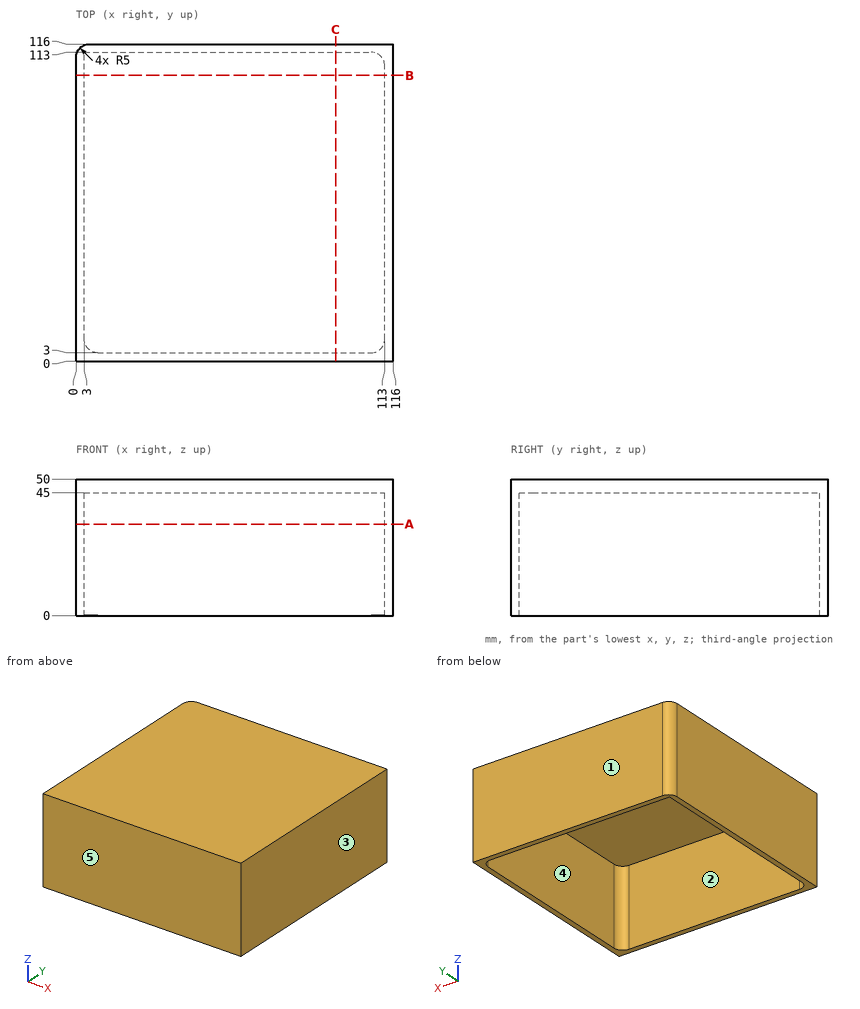
Study the drawing (mm; zero at the part's minimum x, y, z) and answer. A direction names the side the tool comes from. Coordinates: 2 decimals unless noted, no trailing zeros. Loops run counter-clockwise (first coordinate to the right, second up) from the corner with the lowest first, then second, coordinate; pieces in that order, holes last. Notation, with made-up numbers: (75.25, -26) -> (90.25, -26) arc R30 cw to (90.25, 1) -> close; hole circle Ø6 at (65, -11.75). An arc over 180 degrees is marked (long way). Answer in a Markdown table with one row per item. Add a question column.
1. Determine the mould class of the marked faces 1, 2 and 3 for opening direction Y: +Y half, -Y half, draft (parallel to the pull), parting line (faces both ways), or undercut.
2. Consider line 1 (Y direction, x = 87, z = 6); line 2 (Z direction, x = 68.5, y = 90.5). Determine where each line is inside the solid, lowest interval first. Write a range as [from, to].
3. For the marked faces 4 and 5, determine the directions among +Z, -Z, +X, -X, +Y, -Y from which every point of the face is accessible in a straight line to the end or side of a thin tool.
4. A flat-ended cylindrical pin translates along its axis: P1, Ø10, axis at x = 74, y = 20.5, coming from the -Z side. Find the tip coordinate at first contact, or state that the pin passes through.
5. The part is cut by section A-A, the plane z = 33.5. Write down the section's boundary in (x, y).
6. The part is cut by section B-B, the plane y = 104.5. Write down the section's boundary in (x, z).
Answer below:
| question | item | result |
|---|---|---|
| 1 | face 1 | +Y half |
| 1 | face 2 | undercut |
| 1 | face 3 | draft |
| 2 | line 1 | [0, 3], [113, 116] |
| 2 | line 2 | [45, 50] |
| 3 | face 4 | -Z |
| 3 | face 5 | +Z, -Z, +X, -X, -Y |
| 4 | P1 | z = 45 |
| 5 | outline | (0, 0) -> (116, 0) -> (116, 116) -> (5, 116) arc R5 ccw to (0, 111) -> close; hole (3, 8) arc R5 ccw to (8, 3) -> (108, 3) arc R5 ccw to (113, 8) -> (113, 108) arc R5 ccw to (108, 113) -> (3, 113) -> close |
| 6 | outline | (0, 0) -> (3, 0) -> (3, 45) -> (113, 45) -> (113, 0) -> (116, 0) -> (116, 50) -> (0, 50) -> close |
